Design review of the part built by this model. Coordinates are the model's own, in mm. A direction names the side the tool comes from. Coordinates: 2 decimals unless noted, no trailing zeros. Write each loop counter-clockwise with the first axis right and the second up, starting at its lowest first coordinate (ties: lowest second). Pieces come first, ordered by that corner, then holes.
Q1. Mouldability with a two-part tool opening along X and no side actions: class faces 1 (the cylindrical face through (2.401, 0.129, 8.585)), 2 (the cylindrical face through (-1.799, -0.131, 20.115)), 3 (the flat face through (0, -6.45, 3)) as pulls with the +X half, pulls with the -X half, needs draft (parallel to the pull), parting line crosses it, or undercut.
Q2. Machinability: for faces 4 (the flat face through (0, 0, 20.4)), 5 (the flat face through (4.1, -6.2, 0)), 6 (the flat face through (2.1, 0, 14)), 7 (the flat face through (-2.1, 0, 14)), 8 (the flat face through (0, 6.45, 3)), which of the approach directions +Z, -Z, +X, -X, +Y, -Y give a long, thin tool a straight path to every point of the face, cutting with its end or side? Answer none if there is none.
Q3. Take a section at D-D (z = 15.25). Give the boundary of the cut face in (x, y), and give its area (3 significant figures).
Q4. Insertion check: pin 1 (8 mm diameter, centred on y = -1.5, z = 13.5, fed in from -X); pin 2 (5 mm diameter, centred on x = -7, y = -3, fed in from +Z); pin 3 (3 mm diameter, centred on y = -4, z = 9.5, fed in from +X). Each pin has a flat end and moves straight along its axis. Give the tip position at first contact, or say it passes through.
Q5. Take a section at C-C (y = 5.25). Give the boundary of the cut face in (x, z), and give its area (3 significant figures).
Q6. Take a section at B-B (x = 0). Give the boundary of the cut face in (y, z).
Q7. Take a section at A-A (z = 1.5). Give the boundary of the cut face in (x, y), and give its area (3 significant figures).
Q8. For probe 1 along X at (y, z) = (7, 13.5); probe 2 along Z at (x, y) = (7.75, -4); probe 3 along Y at (x, z) = (-5.25, 3.75), list the stretches that pass through material, from the lowest coordinate up.
```python
from build123d import *

# Parameters (mm, degrees)
SKETCH_R        = 9.45
PAD_DEPTH       = 20.4
POCKET_DEPTH    = 12.1
FILLET_R        = 1
POCKET001_DEPTH = 5.3


with BuildPart() as part:
    # Sketch → Pad (new body)
    with BuildSketch(Plane.XY):
        Circle(SKETCH_R)
    extrude(amount=PAD_DEPTH)

    # Sketch001 (on Face3 of Pad) → Pocket (cut)
    with BuildSketch(Plane.XY.offset(20.4)):
        with BuildLine():
            ThreePointArc((-2.100006, 9.213711), (-9.45, 0), (-2.100006, -9.213711))
            Line((-2.100006, 9.213711), (-2.100006, -9.213711))
        make_face()
        with BuildLine():
            ThreePointArc((2.099994, -9.213714), (9.45, 0), (2.099994, 9.213714))
            Line((2.099994, -9.213714), (2.099994, 9.213714))
        make_face()
    extrude(amount=-POCKET_DEPTH, mode=Mode.SUBTRACT)

    # Fillet
    fillet_edges = [part.edges().sort_by_distance(p)[0] for p in [
        (2.099994, 0, 20.4),
        (-2.100006, 0, 20.4),
        (2.099994, 0, 8.3),
        (-2.100006, 0, 8.3),
    ]]
    fillet(fillet_edges, radius=FILLET_R)

    # Sketch002 (on Face5 of Fillet) → Pocket001 (cut)
    with BuildSketch(Plane(origin=(0, 0, 0), x_dir=(1, 0, 0), z_dir=(0, 0, -1))):
        Polygon((-3.723909, 6.45), (-7.447818, 0), (-3.723909, -6.45), (3.723909, -6.45), (7.447818, 0), (3.723909, 6.45), align=None)
    extrude(amount=-POCKET001_DEPTH, mode=Mode.SUBTRACT)


solid = part.part
```
Response:
1. face 1: pulls with the +X half
1. face 2: pulls with the -X half
1. face 3: undercut
2. face 4: +Z, +X, -X, +Y, -Y
2. face 5: -Z, +X, -X, +Y, -Y
2. face 6: +Z, +X, +Y, -Y
2. face 7: +Z, -X, +Y, -Y
2. face 8: -Z
3. outline: (-2.1, -9.21) arc R9.45 ccw to (2.1, -9.21) - (2.1, 9.21) arc R9.45 ccw to (-2.1, 9.21) - close
3. area: 78.7 mm2
4. pin 1: stops at x = -2.1
4. pin 2: stops at z = 8.3
4. pin 3: stops at x = 8.93
5. outline: (-7.86, 0) - (-4.42, 0) - (-4.42, 5.3) - (4.42, 5.3) - (4.42, 0) - (7.86, 0) - (7.86, 8.3) - (3.1, 8.3) arc R1 cw to (2.1, 9.3) - (2.1, 19.4) arc R1 ccw to (1.1, 20.4) - (-1.1, 20.4) arc R1 ccw to (-2.1, 19.4) - (-2.1, 9.3) arc R1 cw to (-3.1, 8.3) - (-7.86, 8.3) - close
5. area: 134 mm2
6. outline: (-9.45, 0) - (-6.45, 0) - (-6.45, 5.3) - (6.45, 5.3) - (6.45, 0) - (9.45, 0) - (9.45, 20.4) - (-9.45, 20.4) - close
7. outline: circle Ø18.9 at (0, 0); hole (-7.45, 0) - (-3.72, -6.45) - (3.72, -6.45) - (7.45, 0) - (3.72, 6.45) - (-3.72, 6.45) - close
7. area: 136 mm2
8. probe 1: x = -2.1 to 2.1
8. probe 2: z = 0 to 8.3
8. probe 3: y = -7.86 to -3.81, 3.81 to 7.86
